Check sheet for the modelled part. Datum: model origin and axes. Units: mm. Face numbers are marked on the shaded views. A direction names the side the tool comes from. Coordinates: 2 decimals unless noted, no trailing zeros. Write each loop counter-clockwise with the first axis right and the second up, starting at its lowest first coordinate (ties: lowest second). Pieces come first, ordered by that corner, then holes. Notation, with made-up numbers: (28, 50) - (45, 50) arc R37 ccw to (45, 86) - close; hole circle Ø4 at (9, 74.25). An arc over 180 degrees is marked (long way). Use one line per item in the form item = value. Start each with the question number.
1. Cross-section at A-A on x = -12. Record the boundary of the cut face in (y, z), then the cut area to 3 significant figures.
2. Go/stop test with flat-tipped pins: pin 1 Ø3 at (x, z) = (-5.5, 62) entering from +Y; pin 2 Ø1.1 at (y, z) = (-43.5, 12) entering from +X; pin 3 Ø12 at (x, z) = (26, 44) entering from +Y; pin 4 Ø2.5 at (x, y) = (0, -42) entering from -Z. Record where each tip stops, or that it passes through.
3. Scan lines: line 1 along Z through (x, y) = (-2, -40); line 2 along Y through (x, z) = (0, 2). Record each from-to range of solid material in increasing order.
4. Cross-section at C-C on y = -25.5. Record the boundary of the cut face in (x, z) (3 decimals), then the cut area to 3 significant figures.
5. Draft check along Y on the marked faces 1, 2, 3 and 4. Enter one of: +Y half, -Y half, draft (parallel to the pull), parting line (faces both ways), or undercut.
6. Tool access check on the marked faces 5, 6 and 7. Record the directions out of +Z, -Z, +X, -X, +Y, -Y that give a thin tool (end or side, any length) a straight path to the whole face; none if there is none.
7. Cross-section at B-B on z = 19.5. Record the boundary of the cut face in (x, y), then the cut area to 3 significant figures.
```python
from build123d import *

# Parameters (mm, degrees)
IZIM1_R                     = 35.2
IZIM1_R_2                   = 1.5
Y_KSEKLIK_EKSTR_ZYON1_DEPTH = 72
Y_KSEKLIK_EKSTR_ZYON2_START = -18
Y_KSEKLIK_EKSTR_ZYON2_DEPTH = 18
KES_EKSTR_ZYON1_DEPTH       = 4.5
DAIRESEL_KAPLAMA1_COUNT     = 4
AYNALAMA1_COPY_1_DEPTH      = 4.5
AYNALAMA1_COPY_2_DEPTH      = 4.5
AYNALAMA1_COPY_3_DEPTH      = 4.5
RADYUS1_R                   = 1


with BuildPart() as part:
    # Çizim1 → Yükseklik-Ekstrüzyon1 (new body)
    with BuildSketch(Plane.XY):
        with BuildLine():
            ThreePointArc((-39.855405506, -10.439667234), (-29.132799385, -29.132799385), (-10.439667234, -39.855405506))
            ThreePointArc((-10.439667234, -39.855405506), (-6.917154276, -41.571669638), (-4.324522349, -44.50968254))
            ThreePointArc((-4.324522349, -44.50968254), (0, -47), (4.324522349, -44.50968254))
            ThreePointArc((4.324522349, -44.50968254), (6.917154276, -41.571669638), (10.439667234, -39.855405506))
            ThreePointArc((10.439667234, -39.855405506), (29.132799385, -29.132799385), (39.855405506, -10.439667234))
            ThreePointArc((39.855405506, -10.439667234), (41.571669638, -6.917154276), (44.50968254, -4.324522349))
            ThreePointArc((44.50968254, -4.324522349), (47, 0), (44.50968254, 4.324522349))
            ThreePointArc((44.50968254, 4.324522349), (41.571669638, 6.917154276), (39.855405506, 10.439667234))
            ThreePointArc((39.855405506, 10.439667234), (29.132799385, 29.132799385), (10.439667234, 39.855405506))
            ThreePointArc((10.439667234, 39.855405506), (6.917154276, 41.571669638), (4.324522349, 44.50968254))
            ThreePointArc((4.324522349, 44.50968254), (0, 47), (-4.324522349, 44.50968254))
            ThreePointArc((-4.324522349, 44.50968254), (-6.917154276, 41.571669638), (-10.439667234, 39.855405506))
            ThreePointArc((-10.439667234, 39.855405506), (-29.132799385, 29.132799385), (-39.855405506, 10.439667234))
            ThreePointArc((-39.855405506, 10.439667234), (-41.571669638, 6.917154276), (-44.50968254, 4.324522349))
            ThreePointArc((-44.50968254, 4.324522349), (-47, 0), (-44.50968254, -4.324522349))
            ThreePointArc((-44.50968254, -4.324522349), (-41.571669638, -6.917154276), (-39.855405506, -10.439667234))
        make_face()
        Circle(IZIM1_R, mode=Mode.SUBTRACT)
        with Locations((-42, 0)):
            Circle(IZIM1_R_2, mode=Mode.SUBTRACT)
        with Locations((0, 42)):
            Circle(IZIM1_R_2, mode=Mode.SUBTRACT)
        with Locations((42, 0)):
            Circle(IZIM1_R_2, mode=Mode.SUBTRACT)
        with Locations((0, -42)):
            Circle(IZIM1_R_2, mode=Mode.SUBTRACT)
    extrude(amount=Y_KSEKLIK_EKSTR_ZYON1_DEPTH)

    # Çizim2 → Yükseklik-Ekstrüzyon2 (add)
    with BuildSketch(Plane.XY.offset(72).offset(Y_KSEKLIK_EKSTR_ZYON2_START)):
        with BuildLine():
            Line((-4, 34.971988791), (-4, 32.958155288))
            ThreePointArc((-4, 32.958155288), (-16.6, 28.752043406), (-26.542599741, 19.943179259))
            Line((-26.542599741, 19.943179259), (-28.286630714, 20.950096011))
            ThreePointArc((-28.286630714, 20.950096011), (-17.6, 30.484094213), (-4, 34.971988791))
        make_face()
        with BuildLine():
            Line((4, 34.971988791), (4, 32.958155288))
            ThreePointArc((4, 32.958155288), (16.6, 28.752043406), (26.542599741, 19.943179259))
            Line((26.542599741, 19.943179259), (28.286630714, 20.950096011))
            ThreePointArc((28.286630714, 20.950096011), (17.6, 30.484094213), (4, 34.971988791))
        make_face()
        with BuildLine():
            Line((32.286630714, 14.02189278), (30.542599741, 13.014976029))
            ThreePointArc((30.542599741, 13.014976029), (33.2, 0), (30.542599741, -13.014976029))
            Line((30.542599741, -13.014976029), (32.286630714, -14.02189278))
            ThreePointArc((32.286630714, -14.02189278), (35.2, 0), (32.286630714, 14.02189278))
        make_face()
        with BuildLine():
            Line((28.286630714, -20.950096011), (26.542599741, -19.943179259))
            ThreePointArc((26.542599741, -19.943179259), (16.6, -28.752043406), (4, -32.958155288))
            Line((4, -32.958155288), (4, -34.971988791))
            ThreePointArc((4, -34.971988791), (17.6, -30.484094213), (28.286630714, -20.950096011))
        make_face()
        with BuildLine():
            Line((-4, -34.971988791), (-4, -32.958155288))
            ThreePointArc((-4, -32.958155288), (-16.6, -28.752043406), (-26.542599741, -19.943179259))
            Line((-26.542599741, -19.943179259), (-28.286630714, -20.950096011))
            ThreePointArc((-28.286630714, -20.950096011), (-17.6, -30.484094213), (-4, -34.971988791))
        make_face()
        with BuildLine():
            Line((-32.286630714, -14.02189278), (-30.542599741, -13.014976029))
            ThreePointArc((-30.542599741, -13.014976029), (-33.2, 0), (-30.542599741, 13.014976029))
            Line((-30.542599741, 13.014976029), (-32.286630714, 14.02189278))
            ThreePointArc((-32.286630714, 14.02189278), (-35.2, 0), (-32.286630714, -14.02189278))
        make_face()
    extrude(amount=Y_KSEKLIK_EKSTR_ZYON2_DEPTH)

    # Çizim3 → Kes-Ekstrüzyon1 (cut)
    with BuildSketch(Plane(origin=(0, 0, 10), x_dir=(-1, 0, 0), z_dir=(0, 0, -1))):
        Polygon((-3.262029021, -42), (-3.262029021, -48), (3.262029021, -48), (3.262029021, -42), (1.63101451, -39.175), (-1.63101451, -39.175), align=None)
    kes_ekstr_zyon1 = extrude(amount=-KES_EKSTR_ZYON1_DEPTH, mode=Mode.SUBTRACT)

    # Dairesel Kaplama1: Kes-Ekstrüzyon1 ×4 about axis
    dairesel_kaplama1_axis = Axis((0, 0, 0), (0, 0, 1))
    for i in range(1, DAIRESEL_KAPLAMA1_COUNT):
        add(kes_ekstr_zyon1.rotate(dairesel_kaplama1_axis, i * 360 / DAIRESEL_KAPLAMA1_COUNT), mode=Mode.SUBTRACT)

    # Aynalama1: Kes-Ekstrüzyon1 across plane
    add(kes_ekstr_zyon1.mirror(Plane(origin=(0, 0, 36), x_dir=(1, 0, 0), z_dir=(0, 0, -1))), mode=Mode.SUBTRACT)

    # Aynalama1 copy 1 sketch → Aynalama1 copy 1 (cut)
    with BuildSketch(Plane(origin=(0, 0, 62), x_dir=(0, -1, 0), z_dir=(0, 0, 1))):
        Polygon((-3.262029021, 42), (-3.262029021, 48), (3.262029021, 48), (3.262029021, 42), (1.63101451, 39.175), (-1.63101451, 39.175), align=None)
    extrude(amount=-AYNALAMA1_COPY_1_DEPTH, mode=Mode.SUBTRACT)

    # Aynalama1 copy 2 sketch → Aynalama1 copy 2 (cut)
    with BuildSketch(Plane.XY.offset(62)):
        Polygon((-3.262029021, 42), (-3.262029021, 48), (3.262029021, 48), (3.262029021, 42), (1.63101451, 39.175), (-1.63101451, 39.175), align=None)
    extrude(amount=-AYNALAMA1_COPY_2_DEPTH, mode=Mode.SUBTRACT)

    # Aynalama1 copy 3 sketch → Aynalama1 copy 3 (cut)
    with BuildSketch(Plane(origin=(0, 0, 62), x_dir=(0, 1, 0), z_dir=(0, 0, 1))):
        Polygon((-3.262029021, 42), (-3.262029021, 48), (3.262029021, 48), (3.262029021, 42), (1.63101451, 39.175), (-1.63101451, 39.175), align=None)
    extrude(amount=-AYNALAMA1_COPY_3_DEPTH, mode=Mode.SUBTRACT)

    # Radyus1
    radyus1_edges = [part.edges().sort_by_distance(p)[0] for p in [
        (4, -32.958155288, 63),
        (26.542599741, -19.943179259, 63),
        (-26.542599741, -19.943179259, 63),
        (-4, -32.958155288, 63),
        (-30.542599741, 13.014976029, 63),
        (-30.542599741, -13.014976029, 63),
        (26.542599741, 19.943179259, 63),
        (4, 32.958155288, 63),
        (-4, 32.958155288, 63),
        (-26.542599741, 19.943179259, 63),
        (30.542599741, -13.014976029, 63),
        (30.542599741, 13.014976029, 63),
    ]]
    fillet(radyus1_edges, radius=RADYUS1_R)


solid = part.part
```
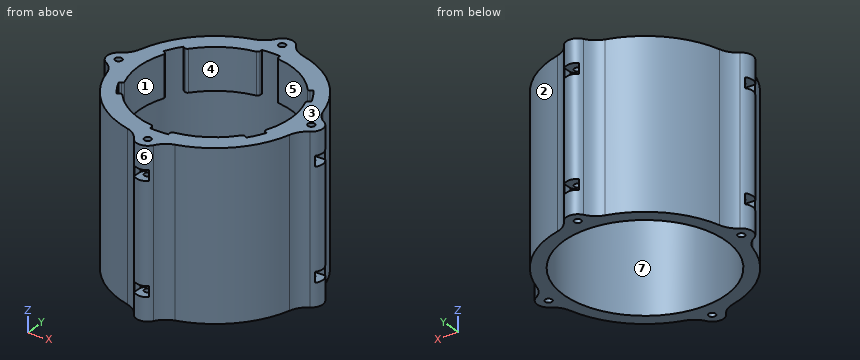
Final values:
q1.outline = (-39.41, 0) - (-33.09, 0) - (-33.09, 54) - (-30.96, 54) - (-30.96, 72) - (-39.41, 72) - close; (30.96, 54) - (33.09, 54) - (33.09, 0) - (39.41, 0) - (39.41, 72) - (30.96, 72) - close
q1.area = 987 mm²
q2.pin_1 = 45
q2.pin_2 = 5.44
q2.pin_3 = 36.02
q2.pin_4 = through
q3.line_1 = 0 to 10, 14.5 to 57.5, 62 to 72
q3.line_2 = -47 to -43.5, -40.5 to -35.2, 35.2 to 40.5, 43.5 to 47
q4.outline = (-32.36, 0) - (-24.265, 0) - (-24.265, 54) - (-21.26, 54) - (-21.26, 72) - (-32.36, 72) - close; (21.26, 54) - (24.265, 54) - (24.265, 0) - (32.36, 0) - (32.36, 72) - (21.26, 72) - close
q4.area = 1,270 mm²
q5.face_1 = undercut
q5.face_2 = +Y half
q5.face_3 = draft
q5.face_4 = undercut
q6.face_5 = +Z, -Z
q6.face_6 = +Z, -Z, -Y
q6.face_7 = -Z
q7.outline = (-44.51, -4.32) arc R10 cw to (-39.86, -10.44) arc R41.2 ccw to (-10.44, -39.86) arc R10 cw to (-4.32, -44.51) arc R5 ccw to (4.32, -44.51) arc R10 cw to (10.44, -39.86) arc R41.2 ccw to (39.86, -10.44) arc R10 cw to (44.51, -4.32) arc R5 ccw to (44.51, 4.32) arc R10 cw to (39.86, 10.44) arc R41.2 ccw to (10.44, 39.86) arc R10 cw to (4.32, 44.51) arc R5 ccw to (-4.32, 44.51) arc R10 cw to (-10.44, 39.86) arc R41.2 ccw to (-39.86, 10.44) arc R10 cw to (-44.51, 4.32) arc R5 ccw to start; hole circle Ø3 at (-42, 0); hole circle Ø70.4 at (0, 0); hole circle Ø3 at (0, -42); hole circle Ø3 at (0, 42); hole circle Ø3 at (42, 0)
q7.area = 1,640 mm²
